from build123d import *

# Parameters (mm, degrees)
SKETCH1_R           = 18
SKETCH1_R_2         = 15.5
BOSS_EXTRUDE1_DEPTH = 3
SKETCH2_R           = 18
SKETCH2_R_2         = 10
BOSS_EXTRUDE2_DEPTH = 1
THREAD2_PITCH       = 1
THREAD2_TO          = 4


with BuildPart() as part:
    # Sketch1 → Boss-Extrude1 (new body)
    with BuildSketch(Plane(origin=(0, 0, 0), x_dir=(1, 0, 0), z_dir=(0, 1, 0))):
        with Locations(Location((0, 0, 0), (0, 0, 270))):
            Circle(SKETCH1_R)
        with Locations(Location((0, 0, 0), (0, 0, 270))):
            Circle(SKETCH1_R_2, mode=Mode.SUBTRACT)
    extrude(amount=BOSS_EXTRUDE1_DEPTH)

    # Sketch2 → Boss-Extrude2 (add)
    with BuildSketch(Plane(origin=(0, 3, 0), x_dir=(1, 0, 0), z_dir=(0, 1, 0))):
        with Locations(Location((0, 0, 0), (0, 0, 270))):
            Circle(SKETCH2_R)
        with Locations(Location((0, 0, 0), (0, 0, 270))):
            Circle(SKETCH2_R_2, mode=Mode.SUBTRACT)
    extrude(amount=BOSS_EXTRUDE2_DEPTH)

    # Thread2: arcs per turn and ends read off the stored shape
    # Thread2: the profile of Thread Profile2 profile screwed along a right-hand helix through 4 turns, 8 arcs to a turn; built about Z, then put on its axis
    thread2_z = Axis((0, 0, 0), (0, 0, 1))
    thread2_corners = [(15.4997, 0, -0.000173205), (16.041265875, 0, 0.312499999), (16.041265875, 0, 0.437499999), (15.4997, 0, 0.750173202)]
    with BuildLine(mode=Mode.PRIVATE) as thread2_profile:
        Line(thread2_corners[0], thread2_corners[1])
        Line(thread2_corners[1], thread2_corners[2])
        Line(thread2_corners[2], thread2_corners[3])
        Line(thread2_corners[3], thread2_corners[0])
    thread2_cap = Face(thread2_profile.wire())
    thread2_turn_angles = [0, 22.5, 45, 67.5, 90, 112.5, 135, 157.5, 180, 202.5, 225, 247.5, 270, 292.5, 315, 337.5, 360]
    thread2_turn_weights = [1, 0.9238795325112867, 1, 0.9238795325112867, 1, 0.9238795325112867, 1, 0.9238795325112867, 1, 0.9238795325112867, 1, 0.9238795325112867, 1, 0.9238795325112867, 1, 0.9238795325112867, 1]
    thread2_turn_rails = [Edge.make_bspline([Vector(p[0], p[1], 0).rotate(thread2_z, thread2_turn_angles[k]) / thread2_turn_weights[k] + Vector(0, 0, p[2] + THREAD2_PITCH * thread2_turn_angles[k] / 360) for k in range(17)], [0, 0, 0, 1, 1, 2, 2, 3, 3, 4, 4, 5, 5, 6, 6, 7, 7, 8, 8, 8], 2, thread2_turn_weights) for p in thread2_corners]
    thread2_turn_sides = [Face.make_surface_from_curves(thread2_turn_rails[p[0]], thread2_turn_rails[p[1]]) for p in [(0, 1), (1, 2), (2, 3), (3, 0)]]
    thread2 = Plane(origin=(0, -1, 0), x_dir=(1, 0, 0), z_dir=(0, 1, 0)) * split(Solid(Shell([*[p.moved(Location((0, 0, THREAD2_PITCH * i))) for i in range(4) for p in thread2_turn_sides], thread2_cap, thread2_cap.rotate(thread2_z, 1440).moved(Location((0, 0, THREAD2_PITCH * 1440 / 360)))])), bisect_by=Plane.XY.offset(THREAD2_TO), keep=Keep.BOTTOM, mode=Mode.PRIVATE)
    add(thread2, mode=Mode.SUBTRACT)


solid = part.part
Here's how the part is built. I have some questions about the finished solid (model axes, mm). Round coordinates to 2 decimals unless told otherwise and drop trailing zeros. Write each loop counter-clockwise with the first axis right and the second up, starting at its lowest first coordinate (ties: lowest second). Pieces come first, ordered by that corner, then holes.
1. I need wall thicknesses on L1, parallel to X at y = 3.6, z = 0; L2, parallel to X at y = 1.35, z = 0.5; L3, parallel to Y at x = 15, z = 1.5. Which ranges of each line are inside material? Lowest first, please.
2. Suppose I cut it at A-A (y = 3.55). List the corners of the cut face in (x, z) for me, and give its area (3 significant figures).
3. If we mould it in two halves opening along X, with no side actions, what happens to faces 1 (the flat face through (-5, 0, -15)), 2 (the cylindrical face through (5.407, 1.972, 17.169)), 3 (the flat face through (-10.5, 3, 0)), 4 (the cylindrical face through (-9.76, 3.49, -2.17))? For each: released by +X, released by -X, zero draft, split by the parting line, or undercut.
4. Will these pins go through, and if not, where does the flat tip stop? pin 1 Ø1 at (x, y) = (-5, 1.5) entering from +Z; pin 2 Ø2 at (x, z) = (5, 8.5) entering from -Y.
Answer sheet:
1. L1: x = -18 to -10, 10 to 18
1. L2: x = -17.99 to -15.49, 16.03 to 17.99
1. L3: y = 3 to 4
2. outline: circle Ø36 at (0, 0); hole circle Ø20 at (0, 0)
2. area: 704 mm2
3. face 1: zero draft
3. face 2: split by the parting line
3. face 3: undercut
3. face 4: undercut
4. pin 1: stops at z = 17.43
4. pin 2: stops at y = 3
